from build123d import *

# Parameters (mm, degrees)
CROQUIS1_R              = 1.5
SALIENTE_EXTRUIR1_DEPTH = 6


with BuildPart() as part:
    # Croquis1 → Saliente-Extruir1 (new body)
    with BuildSketch(Plane.XY):
        with BuildLine():
            Line((-283.764, 132.5), (-132.5, 132.5))
            Line((-132.5, 132.5), (-132.5, 283.764))
            ThreePointArc((-132.5, 283.764), (-127.012352652, 297.012352652), (-113.764, 302.5))
            Line((-113.764, 302.5), (113.764, 302.5))
            ThreePointArc((113.764, 302.5), (127.012352652, 297.012352652), (132.5, 283.764))
            Line((132.5, 283.764), (132.5, 132.5))
            Line((132.5, 132.5), (283.764, 132.5))
            ThreePointArc((283.764, 132.5), (297.012352652, 127.012352652), (302.5, 113.764))
            Line((302.5, 113.764), (302.5, -113.764))
            ThreePointArc((302.5, -113.764), (297.012352652, -127.012352652), (283.764, -132.5))
            Line((283.764, -132.5), (132.5, -132.5))
            Line((132.5, -132.5), (132.5, -283.764))
            ThreePointArc((132.5, -283.764), (127.012352652, -297.012352652), (113.764, -302.5))
            Line((113.764, -302.5), (-113.764, -302.5))
            ThreePointArc((-113.764, -302.5), (-127.012352652, -297.012352652), (-132.5, -283.764))
            Line((-132.5, -283.764), (-132.5, -132.5))
            Line((-132.5, -132.5), (-283.764, -132.5))
            ThreePointArc((-283.764, -132.5), (-297.012352652, -127.012352652), (-302.5, -113.764))
            Line((-302.5, -113.764), (-302.5, 113.764))
            ThreePointArc((-302.5, 113.764), (-297.012352652, 127.012352652), (-283.764, 132.5))
        make_face()
        with Locations((-282.5, 112.5)):
            Circle(CROQUIS1_R, mode=Mode.SUBTRACT)
        with Locations((-282.5, -112.5)):
            Circle(CROQUIS1_R, mode=Mode.SUBTRACT)
        with Locations((-112.5, -282.5)):
            Circle(CROQUIS1_R, mode=Mode.SUBTRACT)
        with Locations((112.5, -282.5)):
            Circle(CROQUIS1_R, mode=Mode.SUBTRACT)
        with Locations((282.5, -112.5)):
            Circle(CROQUIS1_R, mode=Mode.SUBTRACT)
        with Locations((282.5, 112.5)):
            Circle(CROQUIS1_R, mode=Mode.SUBTRACT)
        with Locations((-112.5, 282.5)):
            Circle(CROQUIS1_R, mode=Mode.SUBTRACT)
        with Locations((112.5, 282.5)):
            Circle(CROQUIS1_R, mode=Mode.SUBTRACT)
        Polygon((-278.5, 122.5), (-122.5, 122.5), (-122.5, 278.5), (-108.5, 278.5), (-108.5, 292.5), (108.5, 292.5), (108.5, 278.5), (122.5, 278.5), (122.5, 122.5), (278.5, 122.5), (278.5, 108.5), (292.5, 108.5), (292.5, -108.5), (278.5, -108.5), (278.5, -122.5), (122.5, -122.5), (122.5, -278.5), (108.5, -278.5), (108.5, -292.5), (-108.5, -292.5), (-108.5, -278.5), (-122.5, -278.5), (-122.5, -122.5), (-278.5, -122.5), (-278.5, -108.5), (-292.5, -108.5), (-292.5, 108.5), (-278.5, 108.5), align=None, mode=Mode.SUBTRACT)
    extrude(amount=SALIENTE_EXTRUIR1_DEPTH)


solid = part.part
Source: CAD feature listing. Evaluate the final solid. Frame: model axes, mm. Coordinates: 2 decimals unless noted, no trailing zeros. Loops run counter-clockwise (first coordinate to the right, second up) from the corner with the lowest first, then second, coordinate; pieces in that order, holes last. Notation, with made-up numbers: (57, -8.5) -> (78, -8.5) arc R27 cw to (78, 7.5) -> close; hole circle Ø7 at (45.25, 45.25). An arc over 180 degrees is marked (long way). Answer in a Markdown table with one row per item. Add a question column.
Q1. Section A-A on x = 47.5. Return the cut outline in (y, z), and give its area (3 significant figures).
Q2. Contact query for flat-ended pins moving along their axis: pin 1 Ø2 at (x, z) = (-226.5, 2) entering from -Y; pin 2 Ø1.5 at (x, z) = (200.5, 5) entering from +Y; pin 3 Ø1.8 at (y, z) = (-182.5, 2) entering from -X. Output: stop coordinate, or through.
Q3. Section C-C on z = 1.65. Give the number of separate pieces and of enclosed holes in the cut face, and give its area (3 significant figures).
Q4. Ray query, line 1 along Y through (x, z) = (112.5, 3.75); line 2 along Y through (x, z) = (282.5, 1.7); line 3 along Y through (x, z) = (-169.5, 1.2). Return the intervals inside material, ascending.
Computed values:
| question | item | result |
|---|---|---|
| 1 | outline | (-302.5, 0) -> (-292.5, 0) -> (-292.5, 6) -> (-302.5, 6) -> close; (292.5, 0) -> (302.5, 0) -> (302.5, 6) -> (292.5, 6) -> close |
| 1 | area | 120 mm^2 |
| 2 | pin 1 | stops at y = -132.5 |
| 2 | pin 2 | stops at y = 132.5 |
| 2 | pin 3 | stops at x = -132.5 |
| 3 | separate pieces | 1 |
| 3 | enclosed holes | 9 |
| 3 | area | 24,700 mm^2 |
| 4 | line 1 | y = -302.5 to -284, -281 to -278.5, 278.5 to 281, 284 to 302.5 |
| 4 | line 2 | y = -132.5 to -114, -111 to -108.5, 108.5 to 111, 114 to 132.5 |
| 4 | line 3 | y = -132.5 to -122.5, 122.5 to 132.5 |
